Drawing for the job (mm, zero at the part's lowest x, y, z). Give positions to 0.01 mm unless a question says otherwise; leave off trailing zeros. Order: outer loops, then holes, each group sorted by start corner. A loop starts at its lowest first (then second) coordinate and runs counter-clockwise, first axis right, second up. Notation, with made-up numbers: (16, 13.5) - (21, 13.5) arc R21 ccw to (21, 38.5) - close; hole circle Ø4 at (-32.75, 39.5). An arc over 180 degrees is marked (long way). Use a Markdown table: item, result. Add a question column.
(1) Wall check: line 1 (Z direction, x = 31, y = 1.25); line 2 (X direction, y = 0.9, z = 28.5); line 3 (Z direction, x = 31.5, y = 0.6). Give the ranges that are in metal, low to high.
(2) Slice it at B-B (z = 7.25). Write the cut outline in (x, y).
(3) Slice it at A-A (y = 1.85). Write the cut outline in (x, z) (1 decimal).
(4) Flat gauge pins, fed straight in: pin 1 (1.5 mm diameter, centred on y = 1, z = 13.5, fed in from +X); pin 2 (5 mm diameter, centred on x = 8, z = 12.5, fed in from -Y); pin 3 (0.9 mm diameter, centred on x = 43, y = 1.5, fed in from -Z); pin 4 (2.5 mm diameter, centred on x = 3.64, z = 2.93, fed in from -Y). Where does each tip first touch, or does it go through?
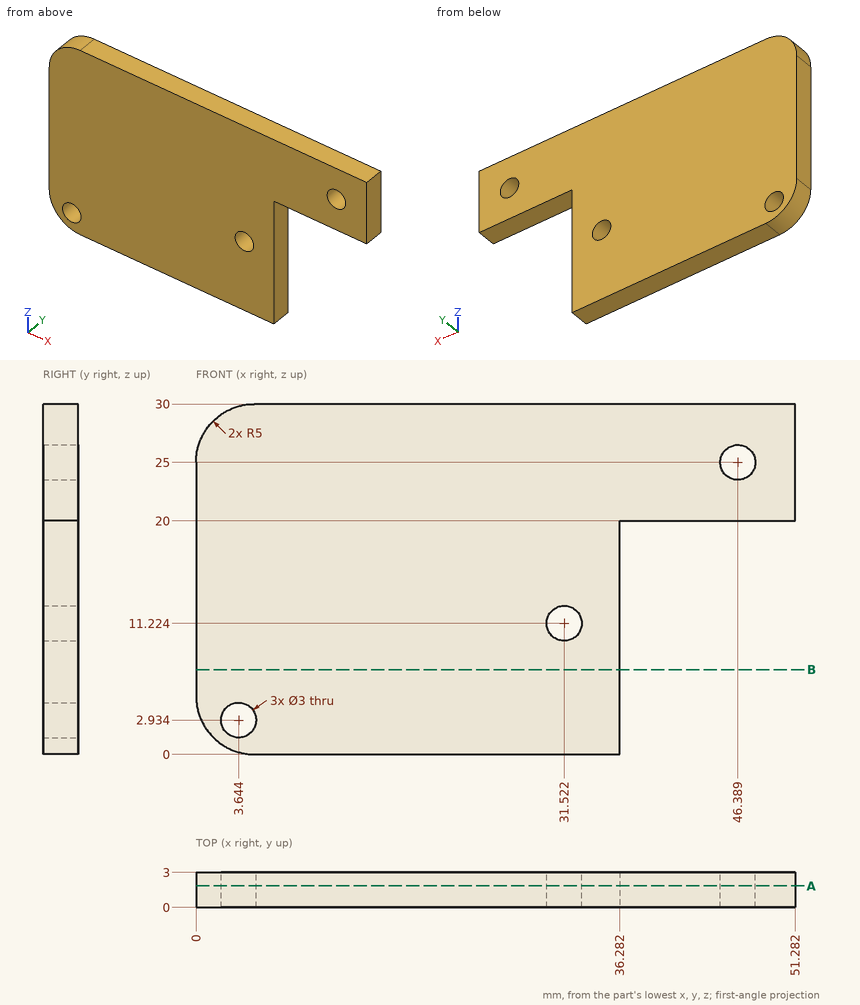
Solution:
| question | item | result |
|---|---|---|
| 1 | line 1 | 0 to 9.82, 12.63 to 30 |
| 1 | line 2 | 1.43 to 51.28 |
| 1 | line 3 | 0 to 9.72, 12.72 to 30 |
| 2 | outline | (0, 0) - (36.28, 0) - (36.28, 3) - (0, 3) - close |
| 3 | outline | (0, 5) arc R5 ccw to (5, 0) - (36.3, 0) - (36.3, 20) - (51.3, 20) - (51.3, 30) - (5, 30) arc R5 ccw to (0, 25) - close; hole circle Ø3 at (3.6, 2.9); hole circle Ø3 at (31.5, 11.2); hole circle Ø3 at (46.4, 25) |
| 4 | pin 1 | x = 36.28 |
| 4 | pin 2 | y = 0 |
| 4 | pin 3 | z = 20 |
| 4 | pin 4 | through |
